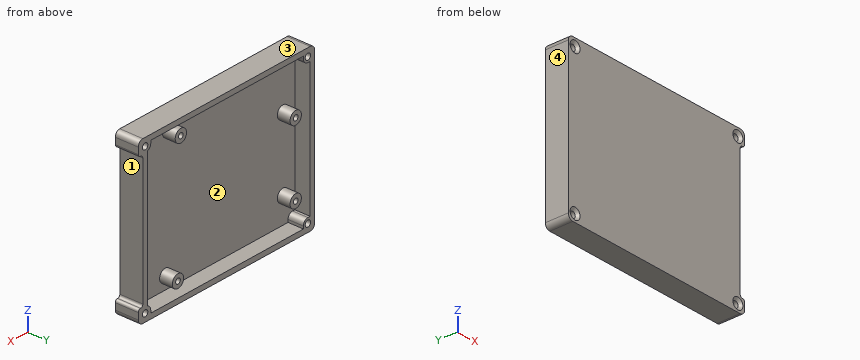
```python
from build123d import *

# Parameters (mm, degrees)
SKETCH1_R                                           = 2.5
BOSS_EXTRUDE1_DEPTH                                 = 5
BOSS_EXTRUDE1_2_DEPTH                               = 5
BOSS_EXTRUDE1_3_DEPTH                               = 5
BOSS_EXTRUDE1_4_DEPTH                               = 5
M2_5_TAPPED_HOLE1_AT_2_COUNT                        = 2
M2_5_TAPPED_HOLE1_AT_2_PITCH                        = 27.94
M2_5_TAPPED_HOLE1_AT_3_COUNT                        = 2
M2_5_TAPPED_HOLE1_AT_3_PITCH                        = 52.317218007
M2_5_TAPPED_HOLE1_AT_4_COUNT                        = 2
M2_5_TAPPED_HOLE1_AT_4_PITCH                        = 66.671976122
BOSS_EXTRUDE2_DEPTH                                 = 3
BOSS_EXTRUDE3_DEPTH                                 = 6
FILLET5_R                                           = 2
CSK_FOR_M2_COUNTERSUNK_FLAT_HEAD_SCREW1_D           = 2.4
CSK_FOR_M2_COUNTERSUNK_FLAT_HEAD_SCREW1_CSINK_D     = 4.4
CSK_FOR_M2_COUNTERSUNK_FLAT_HEAD_SCREW1_CSINK_ANGLE = 90
FILLET6_R                                           = 2
FILLET7_R                                           = 1


# Some blends are built 0.0001 mm under size
with BuildPart() as part:
    # Sketch1 → Boss-Extrude1 (new body)
    with BuildSketch(Plane(origin=(0, 0, 0), x_dir=(1, 0, 0), z_dir=(0, 1, 0))):
        with Locations(Location((-31.75, 19.05, 0), (0, 0, 270))):
            Circle(SKETCH1_R)
    extrude(amount=-BOSS_EXTRUDE1_DEPTH)

    # Sketch13 → M2.5 Tapped Hole1 (revolve, cut)
    with BuildSketch(Plane(origin=(-31.75, 0, -19.05), x_dir=(0, 0, 1), z_dir=(1, 0, 0))):
        Polygon((0, 0), (0, 6.965882135), (1.025, 6.35), (1.025, 0), align=None)
    m2_5_tapped_hole1 = revolve(axis=Axis((-31.75, 6.35, -19.05), (0, -1, 0)), mode=Mode.SUBTRACT)



with BuildPart() as body_2:
    # Sketch1 → Boss-Extrude1 2 (new body)
    with BuildSketch(Plane(origin=(0, 0, 0), x_dir=(1, 0, 0), z_dir=(0, 1, 0))):
        with Locations(Location((-31.75, -8.89, 0), (0, 0, 270))):
            Circle(SKETCH1_R)
    extrude(amount=-BOSS_EXTRUDE1_2_DEPTH)

    # M2.5 Tapped Hole1 at 2: M2.5 Tapped Hole1 ×2
    with Locations(*[(0, 0, i * M2_5_TAPPED_HOLE1_AT_2_PITCH) for i in range(1, M2_5_TAPPED_HOLE1_AT_2_COUNT)]):
        add(m2_5_tapped_hole1, mode=Mode.SUBTRACT)


with BuildPart() as body_3:
    # Sketch1 → Boss-Extrude1 3 (new body)
    with BuildSketch(Plane(origin=(0, 0, 0), x_dir=(1, 0, 0), z_dir=(0, 1, 0))):
        with Locations(Location((20.32, 24.13, 0), (0, 0, 270))):
            Circle(SKETCH1_R)
    extrude(amount=-BOSS_EXTRUDE1_3_DEPTH)

    # M2.5 Tapped Hole1 at 3: M2.5 Tapped Hole1 ×2
    with Locations(*[Vector(0.9952746339256161, 0, -0.097099964285426) * (i * M2_5_TAPPED_HOLE1_AT_3_PITCH) for i in range(1, M2_5_TAPPED_HOLE1_AT_3_COUNT)]):
        add(m2_5_tapped_hole1, mode=Mode.SUBTRACT)


with BuildPart() as body_4:
    # Sketch1 → Boss-Extrude1 4 (new body)
    with BuildSketch(Plane(origin=(0, 0, 0), x_dir=(1, 0, 0), z_dir=(0, 1, 0))):
        with Locations(Location((19.05, -24.13, 0), (0, 0, 270))):
            Circle(SKETCH1_R)
    extrude(amount=-BOSS_EXTRUDE1_4_DEPTH)

    # M2.5 Tapped Hole1 at 4: M2.5 Tapped Hole1 ×2
    with Locations(*[Vector(0.7619393177594593, 0, 0.6476484200955406) * (i * M2_5_TAPPED_HOLE1_AT_4_PITCH) for i in range(1, M2_5_TAPPED_HOLE1_AT_4_COUNT)]):
        add(m2_5_tapped_hole1, mode=Mode.SUBTRACT)


with BuildPart() as part_1:
    add(part.part)

    add(body_2.part)  # Boss-Extrude2 merges body 2

    add(body_3.part)  # Boss-Extrude2 merges body 3

    add(body_4.part)  # Boss-Extrude2 merges body 4
    # Sketch3 → Boss-Extrude2 (add)
    with BuildSketch(Plane.XZ.offset(5)):
        Polygon((-39, 31), (39, 31), (39, 25.5), (37, 25.5), (37, -25.5), (39, -25.5), (39, -31), (-39, -31), align=None)
    extrude(amount=BOSS_EXTRUDE2_DEPTH)

    # Sketch4 → Boss-Extrude3 (add)
    with BuildSketch(Plane(origin=(0, -5, 0), x_dir=(1, 0, 0), z_dir=(0, 1, 0))):
        Polygon((-39, -31), (39, -31), (39, -25.5), (37, -25.5), (37, 25.5), (39, 25.5), (39, 31), (-39, 31), align=None)
        Polygon((-34, -29), (33.5, -29), (33.5, -26), (35, -26), (35, 26), (33.5, 26), (33.5, 29), (-34, 29), (-34, 26), (-37, 26), (-37, -26), (-34, -26), align=None, mode=Mode.SUBTRACT)
    extrude(amount=BOSS_EXTRUDE3_DEPTH)

    # Fillet5
    # the kernel refuses this fillet: 2 mm, written as the material it takes off along each edge
    with BuildSketch(Plane(origin=(33.5, -5, 26), x_dir=(0, 0, 1), z_dir=(0, 1, 0))) as fillet5_piece_1:
        with BuildLine():
            CenterArc((1.936491673, 2), FILLET5_R, 194.477512186, 75.522487814)
            Line((0, 1.5), (-0.038729833, 1.49))
            ThreePointArc((-0.038729833, 1.49), (-0.04, 0.75), (-0.04, 0))
            Line((-0.04, 0), (0, -0.04))
            Line((0, -0.04), (1.936491673, -0.04))
            Line((1.936491673, -0.04), (1.936491673, 0))
        make_face()
    extrude(amount=10.841229183, mode=Mode.SUBTRACT)
    with BuildSketch(Plane(origin=(33.5, -5, -26), x_dir=(1, 0, 0), z_dir=(0, 1, 0))) as fillet5_piece_2:
        with BuildLine():
            CenterArc((2, 1.936491673), FILLET5_R, 180, 75.522487814)
            Line((0, 1.936491673), (-0.04, 1.936491673))
            Line((-0.04, 1.936491673), (-0.04, 0))
            Line((-0.04, 0), (0, -0.04))
            ThreePointArc((0, -0.04), (0.75, -0.04), (1.49, -0.038729833))
            Line((1.49, -0.038729833), (1.5, 0))
        make_face()
    extrude(amount=10.841229183, mode=Mode.SUBTRACT)
    with BuildSketch(Plane(origin=(-34, -5, -26), x_dir=(0, 0, -1), z_dir=(0, 1, 0)), Plane(origin=(-34, -5, 26), x_dir=(-1, 0, 0), z_dir=(0, 1, 0))) as fillet5_piece_3:
        with BuildLine():
            CenterArc((FILLET5_R, FILLET5_R), FILLET5_R, 180, 90)
            Line((0, FILLET5_R), (-FILLET5_R * 0.02, FILLET5_R))
            Line((-FILLET5_R * 0.02, FILLET5_R), (-FILLET5_R * 0.02, -FILLET5_R * 0.02))
            Line((-FILLET5_R * 0.02, -FILLET5_R * 0.02), (FILLET5_R, -FILLET5_R * 0.02))
            Line((FILLET5_R, -FILLET5_R * 0.02), (FILLET5_R, 0))
        make_face()
    extrude(amount=11, mode=Mode.SUBTRACT)

    # CSK for M2 Countersunk Flat Head Screw1 (through all)
    with Locations(Plane(origin=(0, -8, 0), x_dir=(-1, 0, 0), z_dir=(0, -1, 0))):
        with Locations((-36, 28), (36, 28), (36, -28), (-36, -28)):
            CounterSinkHole(CSK_FOR_M2_COUNTERSUNK_FLAT_HEAD_SCREW1_D / 2, CSK_FOR_M2_COUNTERSUNK_FLAT_HEAD_SCREW1_CSINK_D / 2, counter_sink_angle=CSK_FOR_M2_COUNTERSUNK_FLAT_HEAD_SCREW1_CSINK_ANGLE)

    # Fillet6
    fillet6_edges = [part_1.edges().sort_by_distance(p)[0] for p in [
        (39, -3.5, -31),
        (39, -3.5, 31),
        (-39, -3.5, 31),
        (-39, -3.5, -31),
    ]]
    fillet(fillet6_edges, radius=FILLET6_R)

    # Fillet7
    fillet7_edges = [part_1.edges().sort_by_distance(p)[0] for p in [
        (37, -3.5, -25.5),
        (37, -3.5, 25.5),
    ]]
    fillet(fillet7_edges, radius=FILLET7_R)
    fillet7_2_edges = [part_1.edges().sort_by_distance(p)[0] for p in [
        (39, -3.5, -25.5),
        (39, -3.5, 25.5),
    ]]
    fillet(fillet7_2_edges, radius=FILLET7_R - 0.0001)  # a hair under: the kernel refuses the full size


solid = part_1.part
```
Design review of the part built by this model. Coordinates are the model's own, in mm. Face numbers are marked on the shaded views. Give positions to 0.01 mm unless a question says otherwise; leave off trailing zeros. Order: outer loops, then holes, each group sorted by start corner. A loop starts at its lowest first (then second) coordinate and runs counter-clockwise, first axis right, second up. Notation, with made-up numbers: (88.5, -6.5) - (101.5, -6.5) arc R19 cw to (101.5, 5.5) - close; hole circle Ø11 at (-8.5, -26). An arc over 180 degrees is marked (long way). Use a Markdown table: item, result. Add a question column.
(1) Add section A-A on x = 36. Give the boundary of the cut face in (y, z).
(2) Clearance check with flat-ended pins moving along their axes: P1, Ø3, axis at y = -4.5, z = 2.5, coming from the +X side; P2, Ø2.5, axis at x = -31.75, z = 8.89, coming from the +Y side. State where each tip first meets the part, or that it passes through.
(3) Add section B-B on x = -13.5. Give the boundary of the cut face in (y, z).
(4) Mouldability with a two-part tool opening along X and no side actions: class the marked faces 1, 2, 3 and 4 as +X half, -X half, draft (parallel to the pull), parting line (faces both ways), or undercut.
(5) Add section C-C on z = 8.89. Give the boundary of the cut face in (x, y) (3 decimals).
(6) Wall thickness on probe 1 along Z at (x, y) = (36, -5); probe 2 along X at (y, z) = (-1.65, -19.05) (3 decimals); probe 3 along Z at (x, y) = (-36, -2.75): over which ranges is each line inside the solid? List them lowest first. Write a range as [from, to].
(7) Add section D-D on y = -3.5. Give the number of separate pieces and of enclosed holes in the cut face, then the cut area to 3 significant figures.
Report:
| question | item | result |
|---|---|---|
| 1 | outline | (-8, -31) - (1, -31) - (1, -29.2) - (-7, -29.2) - (-8, -30.2) - close; (-8, -25.8) - (-7, -26.8) - (1, -26.8) - (1, 26.8) - (-7, 26.8) - (-8, 25.8) - close; (-8, 30.2) - (-7, 29.2) - (1, 29.2) - (1, 31) - (-8, 31) - close |
| 2 | P1 | stops at x = 37 |
| 2 | P2 | stops at y = 0 |
| 3 | outline | (-8, -31) - (1, -31) - (1, -29) - (-5, -29) - (-5, 29) - (1, 29) - (1, 31) - (-8, 31) - close |
| 4 | face 1 | +X half |
| 4 | face 2 | undercut |
| 4 | face 3 | draft |
| 4 | face 4 | -X half |
| 5 | outline | (-39, -8) - (37, -8) - (37, 1) - (35, 1) - (35, -5) - (-29.25, -5) - (-29.25, 0) - (-30.725, 0) - (-30.725, -5) - (-32.775, -5) - (-32.775, 0) - (-34.25, 0) - (-34.25, -5) - (-37, -5) - (-37, 1) - (-39, 1) - close |
| 6 | probe 1 | z = [-31, -29.2], [-26.8, 26.8], [29.2, 31] |
| 6 | probe 2 | x = [-39, -37], [-34.25, -32.775], [-30.725, -29.25], [35, 37] |
| 6 | probe 3 | z = [-31, -29.2], [-26.8, -26], [26, 26.8], [29.2, 31] |
| 7 | separate pieces | 5 |
| 7 | enclosed holes | 9 |
| 7 | area | 626 mm² |
